Geometry: see drawing. Coordinates: mm, zero at the bounding-box minimum. Give positions to 0.01 mm unless a question says otherwise; leave off trailing zeros. Loops run counter-clockwise (first coordinate to the right, second up) from the corner with the lowest first, then second, coordinate; pieces in that order, holes last. Notation, with made-up numbers: M -31,30.5 L 25,30.5 A34 ccw 25,68.5 Z; hole C -24,-8 d2. An arc over 180 degrees is marked long. Put each result on its own line as item: value.
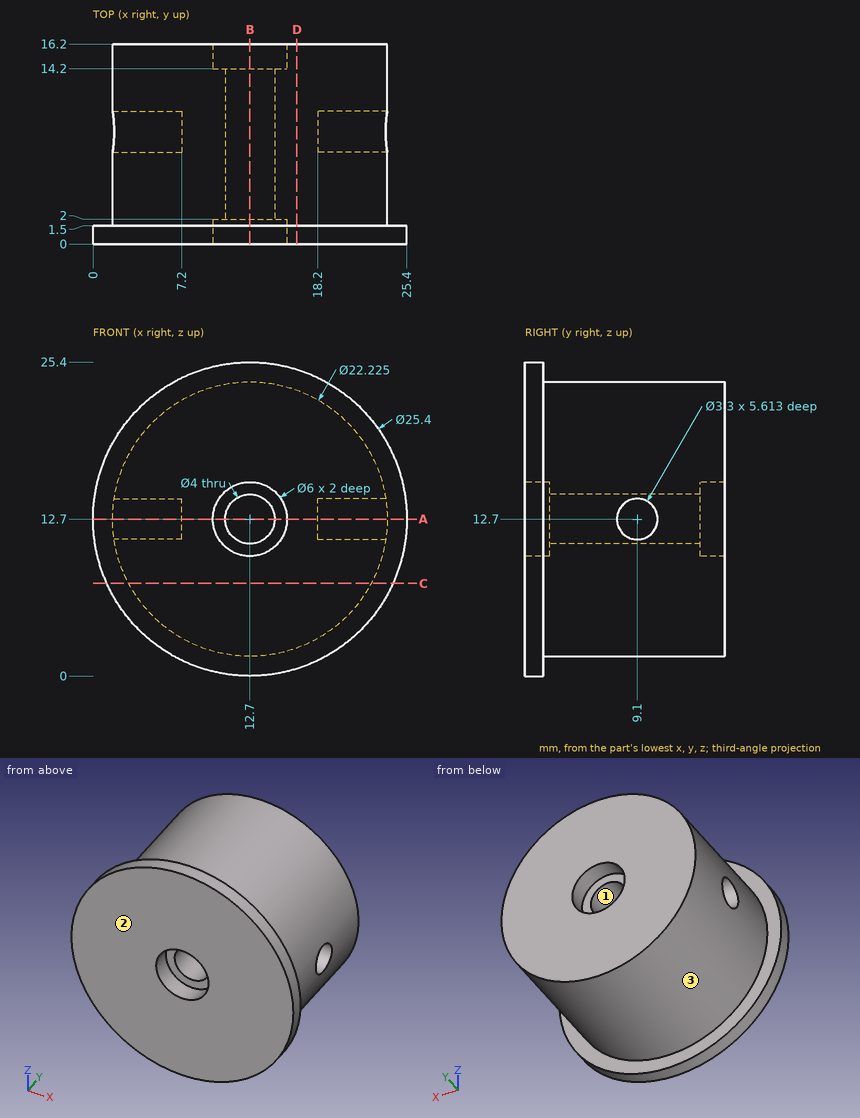
1. Contact query for flat-ended pins moving along their axis: P1, Ø3, axis at y = 6.5, z = 6.5, coming from the -X side; P2, Ø3.5, axis at x = 12.7, z = 12.7, coming from the -Y side; P3, Ø1, axis at y = 10, z = 9, coming from the -X side; P4, Ø3, axis at y = 9.1, z = 12.7, coming from the +X side. Output: stop coordinate, or through.
Found:
P1: x = 2.63
P2: through
P3: x = 2.06
P4: x = 18.2
2. Section query C-C (z = 7.5). Output: boundary loops of the cut face in (x, y).
Found:
outline: M 1.11,0 L 24.29,0 L 24.29,1.5 L 22.52,1.5 L 22.52,16.2 L 2.88,16.2 L 2.88,1.5 L 1.11,1.5 Z
3. Section query A-A (z = 12.7). Output: boundary loops of the cut face in (x, y).
Found:
outline: M 0,0 L 9.7,0 L 9.7,2 L 10.7,2 L 10.7,14.2 L 9.7,14.2 L 9.7,16.2 L 1.59,16.2 L 1.59,10.75 L 7.2,10.75 L 7.2,7.45 L 1.59,7.45 L 1.59,1.5 L 0,1.5 Z; M 14.7,2 L 15.7,2 L 15.7,0 L 25.4,0 L 25.4,1.5 L 23.81,1.5 L 23.81,7.45 L 18.2,7.45 L 18.2,10.75 L 23.81,10.75 L 23.81,16.2 L 15.7,16.2 L 15.7,14.2 L 14.7,14.2 Z
4. Draft query along X for the marked faces 1, 2 and 3. Return one class per face: pulls with the +X half, pulls with the -X half, needs draft (parallel to the pull), parting line crosses it, or undercut.
Found:
face 1: undercut
face 2: needs draft
face 3: parting line crosses it
5. Section query B-B (x = 12.7). Output: boundary loops of the cut face in (y, z).
Found:
outline: M 0,0 L 1.5,0 L 1.5,1.59 L 16.2,1.59 L 16.2,9.7 L 14.2,9.7 L 14.2,10.7 L 2,10.7 L 2,9.7 L 0,9.7 Z; M 0,15.7 L 2,15.7 L 2,14.7 L 14.2,14.7 L 14.2,15.7 L 16.2,15.7 L 16.2,23.81 L 1.5,23.81 L 1.5,25.4 L 0,25.4 Z
6. Material intervals for line 1 (X direction, y = 8.75, z = 12.7); line 2 (Y direction, x = 3.9, z = 12.7); line 3 (X direction, y = 1.25, z = 12.7), sorted ascending. Write a range as from..to.
Found:
line 1: 7.2..10.7, 14.7..18.2
line 2: 0..7.45, 10.75..16.2
line 3: 0..9.7, 15.7..25.4
7. Section query D-D (x = 16.5). Output: boundary loops of the cut face in (y, z), plus the area to 3 significant figures.
Found:
outline: M 0,0.58 L 1.5,0.58 L 1.5,2.26 L 16.2,2.26 L 16.2,23.14 L 1.5,23.14 L 1.5,24.82 L 0,24.82 Z
area: 343 mm^2
